Read the model definition and answer for the solid it produces. Units are mm, in the model's axes. A direction names the side the tool comes from. Give positions to 0.01 mm unless a question says otherwise; leave off trailing zeros. Order: outer loops, then holes, each group sorted by start corner. A loop starts at its lowest first (then second) coordinate and runs counter-clockwise, first axis right, second up. Notation, with made-up numbers: (47, 14.5) - (83, 14.5) arc R16 cw to (83, 40.5) - close; hole circle Ø1 at (-26.75, -6). An arc over 180 degrees is marked (long way). Return JSON: item names as keys, results as strings.
```python
from build123d import *

# Parameters (mm, degrees)
F0_W     = 100
F0_H     = 100
F1_DEPTH = 5
F2_R     = 5
F2_R_2   = 2.5
F3_DEPTH = 5
F6_R     = 5
F6_R_2   = 2.5
F7_DEPTH = 2.5
F8_SIZE  = 2


with BuildPart() as f1:
    # F0 (on Top) → F1 (new body)
    with BuildSketch(Plane.XY):
        Rectangle(F0_W, F0_H)
    extrude(amount=F1_DEPTH)

    # F2 (on face) → F3 (join)
    with BuildSketch(Plane.XY.offset(5)):
        with Locations((-40, 40)):
            Circle(F2_R)
        with Locations((-40, 40)):
            Circle(F2_R_2, mode=Mode.SUBTRACT)
        with Locations((-40, -40)):
            Circle(F2_R)
        with Locations((-40, -40)):
            Circle(F2_R_2, mode=Mode.SUBTRACT)
        with Locations((40, 40)):
            Circle(F2_R)
        with Locations((40, 40)):
            Circle(F2_R_2, mode=Mode.SUBTRACT)
    extrude(amount=F3_DEPTH)

    # F6 (on face) → F7 (join)
    with BuildSketch(Plane.XY.offset(10)):
        with Locations((-40, -40)):
            Circle(F6_R)
        with Locations((-40, -40)):
            Circle(F6_R_2, mode=Mode.SUBTRACT)
        with Locations((40, 40)):
            Circle(F6_R)
        with Locations((40, 40)):
            Circle(F6_R_2, mode=Mode.SUBTRACT)
        with Locations((-40, 40)):
            Circle(F6_R)
        with Locations((-40, 40)):
            Circle(F6_R_2, mode=Mode.SUBTRACT)
    extrude(amount=F7_DEPTH)

    # F8
    f8_edges = [f1.edges().sort_by_distance(p)[0] for p in [
        (-42.5, 40, 12.5),
        (-42.5, -40, 12.5),
        (37.5, 40, 12.5),
    ]]
    chamfer(f8_edges, length=F8_SIZE)


solid = f1.part
```
Q1. Consider L1, parallel to Y at x = -40, z = 8.2; L2, parallel to Y at x = -41, z = 11.5; L3, parallel to Z at x = -30, y = 14. Determine where each line is inside the solid, lowest interval first.
Values:
{"L1": "y = -45 to -42.5, -37.5 to -35, 35 to 37.5, 42.5 to 45", "L2": "y = -44.9 to -43.35, -36.65 to -35.1, 35.1 to 36.65, 43.35 to 44.9", "L3": "z = 0 to 5"}
Q2. Given pin 1 (5.5 mm diameter, centred on x = -41, y = -39, fed in from +Z); pin 2 (4 mm diameter, centred on x = 19, y = -10.5, fed in from +Z); pin 3 (5.5 mm diameter, centred on x = -39.5, y = 39.5, fed in from +Z); pin 4 (6 mm diameter, centred on x = -20.5, y = 17.5, fed in from -Z), each flat-ended and moving along its own axis, determine where each tip first touches the part or whether it passes through.
Values:
{"pin 1": "stops at z = 12.16", "pin 2": "stops at z = 5", "pin 3": "stops at z = 11.46", "pin 4": "stops at z = 0"}
Q3. A cutting plane is placed at B-B (y = 40). Write down the section's boundary in (x, z).
Values:
{"outline": "(-50, 0) - (50, 0) - (50, 5) - (45, 5) - (45, 12.5) - (44.5, 12.5) - (42.5, 10.5) - (42.5, 5) - (37.5, 5) - (37.5, 10.5) - (35.5, 12.5) - (35, 12.5) - (35, 5) - (-35, 5) - (-35, 12.5) - (-35.5, 12.5) - (-37.5, 10.5) - (-37.5, 5) - (-42.5, 5) - (-42.5, 10.5) - (-44.5, 12.5) - (-45, 12.5) - (-45, 5) - (-50, 5) - close"}
Q4. A cutting plane is placed at C-C (x = 40). Write down the section's boundary in (y, z), and give its area (4 significant figures).
Values:
{"outline": "(-50, 0) - (50, 0) - (50, 5) - (45, 5) - (45, 12.5) - (44.5, 12.5) - (42.5, 10.5) - (42.5, 5) - (37.5, 5) - (37.5, 10.5) - (35.5, 12.5) - (35, 12.5) - (35, 5) - (-50, 5) - close", "area": "533.5 mm²"}
Q5. A cutting plane is placed at A-A (z = 8.25). Write down the section's boundary in (x, y), and give its area (3 significant figures).
Values:
{"outline": "circle Ø10 at (-40, -40); circle Ø10 at (-40, 40); circle Ø10 at (40, 40); hole circle Ø5 at (-40, -40); hole circle Ø5 at (-40, 40); hole circle Ø5 at (40, 40)", "area": "177 mm²"}
Q6. Determine the mould class of faces 3 (the cylindrical face through (-37.69, 39.04, 7.71)), 4 (the flat face through (-1, 50, 2)), 5 (the cylindrical face through (-45, -40, 9)), 6 (the flat face through (-50, -1, 2)) for opening direction X: released by +X, released by -X, zero draft, split by the parting line, or undercut.
Values:
{"face 3": "undercut", "face 4": "zero draft", "face 5": "split by the parting line", "face 6": "released by -X"}
Q7. A cutting plane is placed at D-D (y = -40). Write down the section's boundary in (x, z), and give its area (4 significant figures).
Values:
{"outline": "(-50, 0) - (50, 0) - (50, 5) - (-35, 5) - (-35, 12.5) - (-35.5, 12.5) - (-37.5, 10.5) - (-37.5, 5) - (-42.5, 5) - (-42.5, 10.5) - (-44.5, 12.5) - (-45, 12.5) - (-45, 5) - (-50, 5) - close", "area": "533.5 mm²"}
Q8. For faces 1 (the flat face through (50, -1, 2)), 2 (the flat face through (40, 40, 5)), determine the directions among +Z, -Z, +X, -X, +Y, -Y from which every point of the face is accessible in a straight line to the end or side of a thin tool.
Values:
{"face 1": "+Z, -Z, +X, +Y, -Y", "face 2": "+Z"}
